Source: CAD feature listing. Evaluate the final solid. Frame: model axes, mm. Coordinates: 2 decimals unless noted, no trailing zeros. Loops run counter-clockwise (first coordinate to the right, second up) from the corner with the lowest first, then second, coordinate; pieces in that order, holes last. Notation, with made-up numbers: (30.5, 55) -> (63.5, 55) arc R30 ccw to (63.5, 91) -> close; hole circle Ø11 at (66, 57). An arc over 180 degrees is marked (long way). One line per question, with ' | ' between items. Start each with the question number.
```python
from build123d import *

# Parameters (mm, degrees)
EXTRUDE1_DEPTH = 3
CHAMFER1_SIZE  = 0.25


with BuildPart() as part:
    # Sketch1 → Extrude1 (new body)
    with BuildSketch(Plane.XY):
        with BuildLine():
            Line((0, 2.5), (-9, 2.5))
            ThreePointArc((-9, 2.5), (-11.5, 0), (-9, -2.5))
            Line((-9, -2.5), (0, -2.5))
            ThreePointArc((0, -2.5), (2.5, 0), (0, 2.5))
        make_face()
    extrude(amount=EXTRUDE1_DEPTH)

    # Chamfer1
    chamfer1_edges = [part.edges().sort_by_distance(p)[0] for p in [
        (-11.5, 0, 3),
        (-4.5, -2.5, 3),
        (2.5, 0, 3),
        (-4.5, -2.5, 0),
        (-11.5, 0, 0),
        (-4.5, 2.5, 0),
        (2.5, 0, 0),
        (-4.5, 2.5, 3),
    ]]
    chamfer(chamfer1_edges, length=CHAMFER1_SIZE)


solid = part.part
```
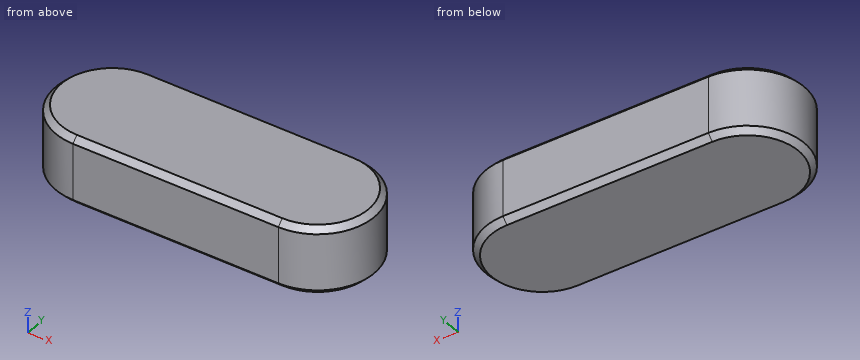
(1) Ray query, L1, parallel to X at y = -1.05, z = 2.7; L2, parallel to X at y = 0.8, z = 0.9; L3, parallel to Y at x = -10.5, z = 1.85. Return the intervals inside material, ascending.
(2) Contact query for flat-ended pins moving along their axis: pin 1 Ø1 at (y, z) = (0.5, 0.5) entering from +X; pin 2 Ø1.5 at (x, z) = (1, 1) entering from +Y. Output: stop coordinate, or through.
(3) Cut plane A-A, the plane z = 0.75. Return the cut outline in (x, y).
Here are the results:
1) L1: x = -11.27 to 2.27 | L2: x = -11.37 to 2.37 | L3: y = -2 to 2
2) pin 1: stops at x = 2.5 | pin 2: stops at y = 2.49
3) outline: (-9, -2.5) -> (0, -2.5) arc R2.5 ccw to (0, 2.5) -> (-9, 2.5) arc R2.5 ccw to start
